Could you check a few things on this drawing? It's one solid part, dimensions in mm from its lowest x, y, z. Give positions to 0.01 mm unless a question says otherwise; leave off trailing zeros. Write each loop counter-clockwise with the first axis right and the second up, starting at its lowest first coordinate (ties: lowest second). Pieces come first, ordered by that corner, then holes. Notation, with made-up numbers: M 89,31.5 L 107,31.5 A24 cw 107,44.5 Z; hole C 71.25,-2 d6. An arc over 180 degrees is marked long. Answer as CSV lines item,"result". Start each with the question number.
Q1. For pin 1 (6 mm diameter, centred on x = 20.5, y = 23.5, fed in from -Z); pin 2 (12 mm diameter, centred on x = 18.5, y = 29.5, fed in from -Z) (3 decimals); pin 3 (1 mm diameter, centred on x = 33, y = 28, fed in from -Z), each with a flat end and sliding along its axis, tell me the tip position at first contact or that it passes through.
Q2. Thinking about a two-plate mould opening in Z: for the marked faces 1, 2 and 3, which applies, +Z half, -Z half, draft (parallel to the pull), parting line (faces both ways), or undercut?
Q3. If I drill on line 1 along Z through (x, y) = (31, 17); line 2 along Z through (x, y) = (32, 30); line 3 along X through (y, z) = (7, 62.5), over which ranges is the centre line in solid material (lowest first)?
Q4. Suppose I cut it at A-A (x = 35). Write out the boundary of the cut face in (y, z).
Q5. Suppose I cut it at B-B (y = 34.5). Write out the boundary of the cut face in (x, z).
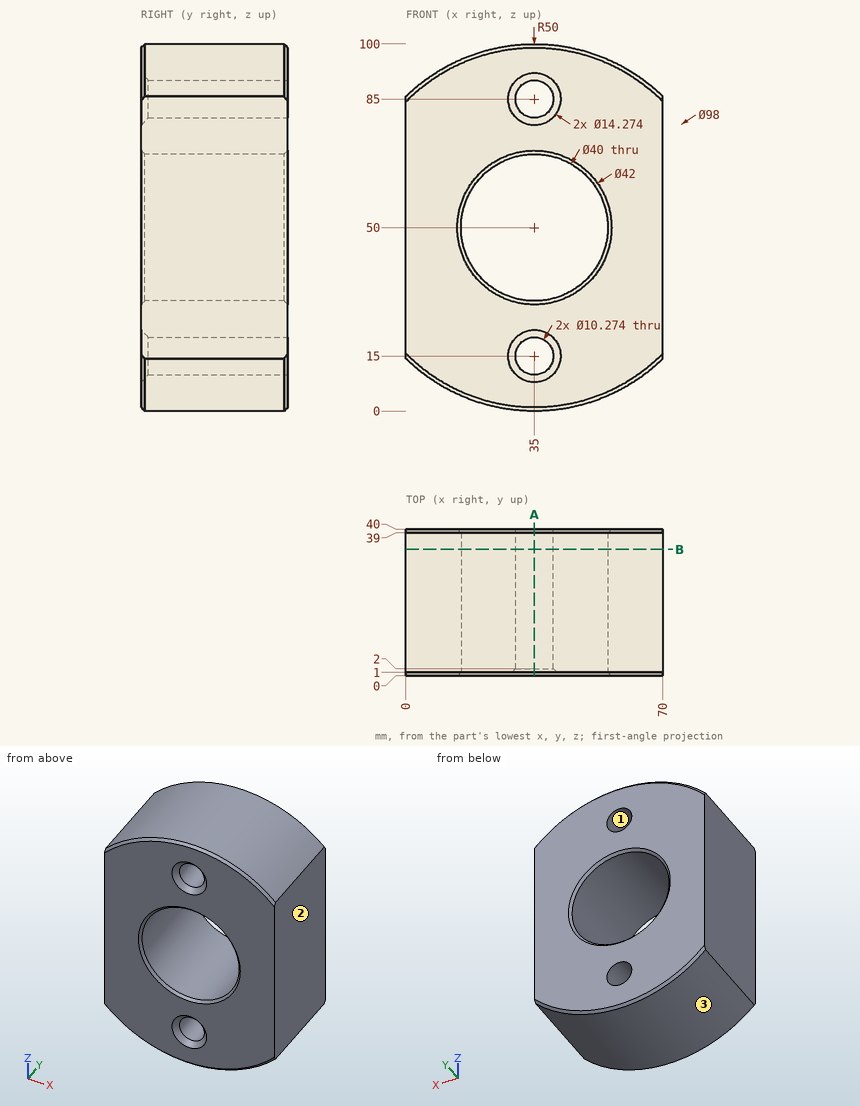
Resolved:
1,pin 1,"z = 1.34"
1,pin 2,"z = 1.115"
1,pin 3,"z = 0.02"
2,face 1,"undercut"
2,face 2,"draft"
2,face 3,"-Z half"
3,line 1,"0.16 to 11.78, 18.22 to 30.4, 69.6 to 81.78, 88.22 to 99.84"
3,line 2,"0.09 to 10.83, 19.17 to 30.23, 69.77 to 80.83, 89.17 to 99.91"
3,line 3,"0 to 19.39, 50.61 to 70"
4,outline,"M 0,1 L 1,0 L 39,0 L 40,1 L 40,9.86 L 2,9.86 L 0,7.86 Z; M 0,22.14 L 2,20.14 L 40,20.14 L 40,29 L 39,30 L 1,30 L 0,29 Z; M 0,71 L 1,70 L 39,70 L 40,71 L 40,79.86 L 2,79.86 L 0,77.86 Z; M 0,92.14 L 2,90.14 L 40,90.14 L 40,99 L 39,100 L 1,100 L 0,99 Z"
5,outline,"M 0,14.29 A50 ccw 70,14.29 L 70,85.71 A50 ccw 0,85.71 Z; hole C 35,50 d40; hole C 35,15 d10.27; hole C 35,85 d10.27"
